CAD build for the part. Positions are in the model's coordinates, mm. A direction names the side the tool comes from. Round coordinates to 2 decimals unless told otherwise and drop trailing zeros. Loops run counter-clockwise (first coordinate to the right, second up) from the corner with the lowest first, then second, coordinate; pieces in that order, holes last. Notation, with made-up numbers: M -27.5,50.25 L -3.5,50.25 A19 cw -3.5,87.25 Z; hole C 24.25,58 d9. An arc over 180 degrees is marked long. Use a Markdown table: item, result. Add a question column.
(1) Flat gauge pins, fed straight in: P1, Ø1.9, axis at x = -57.5, z = 1, coming from the +Y side; P2, Ø1.2, axis at y = -17.5, z = 2, coming from the +X side; P3, Ø0.9, axis at y = -23, z = 1.5, coming from the +X side. Where does each tip first touch, or does it go through?
(2) Two-plate mould, pull along Y, no slides. Class faces 1 (the face through (-58, -4.354, 2)), 2 (the face through (-60.962, -38, 2)), 3 (the face through (-54, -21.854, 2)): released by +Y, released by -Y, zero draft, split by the parting line, or undercut.
(3) Band-saw the part on B-B, the plane z = 0.85. Give the number of separate pieces and of enclosed holes in the cut face, and give its area (3 significant figures).
(4) Which spindle directions (+Z, -Z, +X, -X, +Y, -Y) get a long thin tool onto all of the face, cutting with end or side? Do faces 4 (the face through (-48, 8.146, 2)), 5 (the face through (-55.962, 20, 2)), 6 (the face through (18, 5.146, 2)), 7 (the face through (6.1, -10.2, 2)). Say none if no direction does.
(5) Band-saw the part on A-A, the plane y = 12. Write the cut outline in (x, z), and give its area (3 significant figures).
(6) Wall check: L1, parallel to Y at x = -56, z = 2.25; L2, parallel to Y at x = 19, z = 0.75; L3, parallel to Y at x = -65, z = 1.3. Give the ranges that are in metal, low to high.
from build123d import *

# Parameters (mm, degrees)
SKETCH_1_R      = 3
SKETCH_1_R_2    = 2
SKETCH_1_R_3    = 1.25
EXTRUDE_2_DEPTH = 4
SKETCH_4_W      = 110
SKETCH_4_H      = 6
EXTRUDE_3_DEPTH = 4
FILLET_1_R      = 1.3


with BuildPart() as part:
    # 草图1 → 凸台-拉伸2 (new body)
    with BuildSketch(Plane.XY):
        with BuildLine():
            Line((26.037512023, -61.503506411), (-55.962487977, -61.503506411))
            Line((-55.962487977, -61.503506411), (-55.962487977, -54.853506411))
            Line((-55.962487977, -54.853506411), (-51.962487977, -54.853506411))
            Line((-51.962487977, -54.853506411), (-51.962487977, -56.203506411))
            Line((-51.962487977, -56.203506411), (-49.262487977, -56.203506411))
            Line((-49.262487977, -56.203506411), (-49.262487977, -54.853506411))
            Line((-49.262487977, -54.853506411), (-46.562487977, -54.853506411))
            Line((-46.562487977, -54.853506411), (-46.562487977, -51.853506411))
            Line((-46.562487977, -51.853506411), (-49.262487977, -51.853506411))
            Line((-49.262487977, -51.853506411), (-49.262487977, -50.503506411))
            Line((-49.262487977, -50.503506411), (-51.962487977, -50.503506411))
            Line((-51.962487977, -50.503506411), (-51.962487977, -51.853506411))
            Line((-51.962487977, -51.853506411), (-55.962487977, -51.853506411))
            Line((-55.962487977, -51.853506411), (-55.962487977, -42.353506411))
            Line((-55.962487977, -42.353506411), (-60.962487977, -42.353506411))
            Line((-60.962487977, -42.353506411), (-60.962487977, -34.353506411))
            Line((-60.962487977, -34.353506411), (-55.962487977, -34.353506411))
            Line((-55.962487977, -34.353506411), (-55.962487977, -24.853506411))
            Line((-55.962487977, -24.853506411), (-51.962487977, -24.853506411))
            Line((-51.962487977, -24.853506411), (-51.962487977, -26.203506411))
            Line((-51.962487977, -26.203506411), (-49.262487977, -26.203506411))
            Line((-49.262487977, -26.203506411), (-49.262487977, -24.853506411))
            Line((-49.262487977, -24.853506411), (-46.562487977, -24.853506411))
            Line((-46.562487977, -24.853506411), (-46.562487977, -21.853506411))
            Line((-46.562487977, -21.853506411), (-49.262487977, -21.853506411))
            Line((-49.262487977, -21.853506411), (-49.262487977, -20.503506411))
            Line((-49.262487977, -20.503506411), (-51.962487977, -20.503506411))
            Line((-51.962487977, -20.503506411), (-51.962487977, -21.853506411))
            Line((-51.962487977, -21.853506411), (-55.962487977, -21.853506411))
            Line((-55.962487977, -21.853506411), (-55.962487977, -12.353506411))
            Line((-55.962487977, -12.353506411), (-60.962487977, -12.353506411))
            Line((-60.962487977, -12.353506411), (-60.962487977, -4.353506411))
            Line((-60.962487977, -4.353506411), (-55.962487977, -4.353506411))
            Line((-55.962487977, -4.353506411), (-55.962487977, 5.146493589))
            Line((-55.962487977, 5.146493589), (-51.962487977, 5.146493589))
            Line((-51.962487977, 5.146493589), (-51.962487977, 3.796493589))
            Line((-51.962487977, 3.796493589), (-49.262487977, 3.796493589))
            Line((-49.262487977, 3.796493589), (-49.262487977, 5.146493589))
            Line((-49.262487977, 5.146493589), (-46.562487977, 5.146493589))
            Line((-46.562487977, 5.146493589), (-46.562487977, 8.146493589))
            Line((-46.562487977, 8.146493589), (-49.262487977, 8.146493589))
            Line((-49.262487977, 8.146493589), (-49.262487977, 9.496493589))
            Line((-49.262487977, 9.496493589), (-51.962487977, 9.496493589))
            Line((-51.962487977, 9.496493589), (-51.962487977, 8.146493589))
            Line((-51.962487977, 8.146493589), (-55.962487977, 8.146493589))
            Line((-55.962487977, 8.146493589), (-55.962487977, 23.496493589))
            Line((-55.962487977, 23.496493589), (-55.962487977, 31.722989041))
            ThreePointArc((-55.962487977, 31.722989041), (-14.962487977, 51.269592797), (26.037512023, 31.722989041))
            Line((26.037512023, 31.722989041), (26.037512023, 23.496493589))
            Line((26.037512023, 23.496493589), (26.037512023, 8.146493589))
            Line((26.037512023, 8.146493589), (22.037512023, 8.146493589))
            Line((22.037512023, 8.146493589), (22.037512023, 9.496493589))
            Line((22.037512023, 9.496493589), (19.337512023, 9.496493589))
            Line((19.337512023, 9.496493589), (19.337512023, 8.146493589))
            Line((19.337512023, 8.146493589), (16.637512023, 8.146493589))
            Line((16.637512023, 8.146493589), (16.637512023, 5.146493589))
            Line((16.637512023, 5.146493589), (19.337512023, 5.146493589))
            Line((19.337512023, 5.146493589), (19.337512023, 3.796493589))
            Line((19.337512023, 3.796493589), (22.037512023, 3.796493589))
            Line((22.037512023, 3.796493589), (22.037512023, 5.146493589))
            Line((22.037512023, 5.146493589), (26.037512023, 5.146493589))
            Line((26.037512023, 5.146493589), (26.037512023, -4.353506411))
            Line((26.037512023, -4.353506411), (31.037512023, -4.353506411))
            Line((31.037512023, -4.353506411), (31.037512023, -12.353506411))
            Line((31.037512023, -12.353506411), (26.037512023, -12.353506411))
            Line((26.037512023, -12.353506411), (26.037512023, -21.853506411))
            Line((26.037512023, -21.853506411), (22.037512023, -21.853506411))
            Line((22.037512023, -21.853506411), (22.037512023, -20.503506411))
            Line((22.037512023, -20.503506411), (19.337512023, -20.503506411))
            Line((19.337512023, -20.503506411), (19.337512023, -21.853506411))
            Line((19.337512023, -21.853506411), (16.637512023, -21.853506411))
            Line((16.637512023, -21.853506411), (16.637512023, -24.853506411))
            Line((16.637512023, -24.853506411), (19.337512023, -24.853506411))
            Line((19.337512023, -24.853506411), (19.337512023, -26.203506411))
            Line((19.337512023, -26.203506411), (22.037512023, -26.203506411))
            Line((22.037512023, -26.203506411), (22.037512023, -24.853506411))
            Line((22.037512023, -24.853506411), (26.037512023, -24.853506411))
            Line((26.037512023, -24.853506411), (26.037512023, -34.353506411))
            Line((26.037512023, -34.353506411), (31.037512023, -34.353506411))
            Line((31.037512023, -34.353506411), (31.037512023, -42.353506411))
            Line((31.037512023, -42.353506411), (26.037512023, -42.353506411))
            Line((26.037512023, -42.353506411), (26.037512023, -51.853506411))
            Line((26.037512023, -51.853506411), (22.037512023, -51.853506411))
            Line((22.037512023, -51.853506411), (22.037512023, -50.503506411))
            Line((22.037512023, -50.503506411), (19.337512023, -50.503506411))
            Line((19.337512023, -50.503506411), (19.337512023, -51.853506411))
            Line((19.337512023, -51.853506411), (16.637512023, -51.853506411))
            Line((16.637512023, -51.853506411), (16.637512023, -54.853506411))
            Line((16.637512023, -54.853506411), (19.337512023, -54.853506411))
            Line((19.337512023, -54.853506411), (19.337512023, -56.203506411))
            Line((19.337512023, -56.203506411), (22.037512023, -56.203506411))
            Line((22.037512023, -56.203506411), (22.037512023, -54.853506411))
            Line((22.037512023, -54.853506411), (26.037512023, -54.853506411))
            Line((26.037512023, -54.853506411), (26.037512023, -61.503506411))
        make_face()
        with Locations((-14.962487977, -25.253506411)):
            Circle(SKETCH_1_R, mode=Mode.SUBTRACT)
        with Locations((4.523083608, -12.753506411)):
            Circle(SKETCH_1_R, mode=Mode.SUBTRACT)
        with Locations((-14.962487977, -1.503506411)):
            Circle(SKETCH_1_R_2, mode=Mode.SUBTRACT)
        with Locations((-35.530591317, 10.371493589)):
            Circle(SKETCH_1_R, mode=Mode.SUBTRACT)
        with Locations((-34.448059562, -12.753506411)):
            Circle(SKETCH_1_R, mode=Mode.SUBTRACT)
        with Locations((5.605615363, 10.371493589)):
            Circle(SKETCH_1_R, mode=Mode.SUBTRACT)
        with Locations((-14.962487977, 20.996493589)):
            Circle(SKETCH_1_R, mode=Mode.SUBTRACT)
        with Locations((18.271530739, -34.737525127)):
            Circle(SKETCH_1_R_2, mode=Mode.SUBTRACT)
        with Locations((-14.962487977, -48.503506411)):
            Circle(SKETCH_1_R_2, mode=Mode.SUBTRACT)
        with Locations((-48.196506692, -34.737525127)):
            Circle(SKETCH_1_R_2, mode=Mode.SUBTRACT)
        with Locations((-48.196506692, 31.730512305)):
            Circle(SKETCH_1_R_2, mode=Mode.SUBTRACT)
        with Locations((-14.962487977, 45.496493589)):
            Circle(SKETCH_1_R_2, mode=Mode.SUBTRACT)
        with Locations((18.271530739, 31.730512305)):
            Circle(SKETCH_1_R_2, mode=Mode.SUBTRACT)
        with Locations((-14.962487977, 7.996493589)):
            Circle(SKETCH_1_R_3, mode=Mode.SUBTRACT)
        with Locations((-6.735246641, -6.253506411)):
            Circle(SKETCH_1_R_3, mode=Mode.SUBTRACT)
        with Locations((-23.189729313, -6.253506411)):
            Circle(SKETCH_1_R_3, mode=Mode.SUBTRACT)
    extrude(amount=EXTRUDE_2_DEPTH)

    # 草图4 → 凸台-拉伸3 (add)
    with BuildSketch(Plane.XY.offset(4)):
        with Locations((-14.962487977, -64.503506411)):
            Rectangle(SKETCH_4_W, SKETCH_4_H)
    extrude(amount=-EXTRUDE_3_DEPTH)

    # 圆角1
    fillet_1_edges = [part.edges().sort_by_distance(p)[0] for p in [
        (-60.962487977, -42.353506411, 2),
        (-60.962487977, -34.353506411, 2),
        (-60.962487977, -12.353506411, 2),
        (-60.962487977, -4.353506411, 2),
        (31.037512023, -4.353506411, 2),
        (31.037512023, -12.353506411, 2),
        (31.037512023, -34.353506411, 2),
        (31.037512023, -42.353506411, 2),
    ]]
    fillet(fillet_1_edges, radius=FILLET_1_R)


solid = part.part
Return value:
| question | item | result |
|---|---|---|
| 1 | P1 | y = -4.35 |
| 1 | P2 | x = 26.04 |
| 1 | P3 | x = 16.64 |
| 2 | face 1 | released by +Y |
| 2 | face 2 | zero draft |
| 2 | face 3 | undercut |
| 3 | separate pieces | 1 |
| 3 | enclosed holes | 16 |
| 3 | area | 9,090 mm^2 |
| 4 | face 4 | +Z, -Z, -X |
| 4 | face 5 | +Z, -Z, -X, +Y |
| 4 | face 6 | +Z, -Z, +X |
| 4 | face 7 | +Z, -Z |
| 5 | outline | M -55.96,0 L -38.05,0 L -38.05,4 L -55.96,4 Z; M -33.01,0 L 3.09,0 L 3.09,4 L -33.01,4 Z; M 8.13,0 L 26.04,0 L 26.04,4 L 8.13,4 Z |
| 5 | area | 288 mm^2 |
| 6 | L1 | -67.5 to -61.5, -42.35 to -34.35, -12.35 to -4.35 |
| 6 | L2 | -67.5 to -54.85, -51.85 to -36.6, -32.87 to -24.85, -21.85 to 5.15, 8.15 to 29.87, 33.59 to 38.89 |
| 6 | L3 | -67.5 to -61.5 |
